Geometry: final body of the model. Coordinates: model frame, mm. Give positions to 0.01 mm unless a question says otherwise; leave off trailing zeros. Order: outer loops, then holes, each group sorted by start corner. A loop starts at its lowest first (then second) coordinate and runs counter-clockwise, first axis right, second up. Notation, with made-up numbers: (54, 9) -> (64, 9) arc R14 cw to (64, 24) -> close; hole circle Ø1 at (-5, 83.25). An arc over 180 degrees is marked (long way). Write item = value, one per line.
Autodesk Inventor part; units mm, degrees
ref_plane "Work Plane1" through (5, 2.5, 0) normal (0, 1, 0) x (-1, 0, 0)
ref_plane "YZ Plane" through (0, 0, 0) normal (1, 0, 0) x (0, 1, 0)
ref_plane "XY Plane" through (0, 0, 0) normal (0, 0, 1) x (1, 0, 0)
sketch "Sketch1" plane through (0, 0, 0) normal (0, 0, 1) x (1, 0, 0)
  line L0 (0, 0) -> (51.053, 0) construction
  line L1 (0, 0) -> (0, 2.5)
  line L2 (0, 2.5) -> (10, 2.5)
  line L3 (10, 2.5) -> (10, 4)
  line L4 (10, 4) -> (22, 4)
  line L5 (22, 4) -> (22, 0)
  line L6 (22, 0) -> (0, 0)
  dimension "d0" = 5
  dimension "d1" = 8
  dimension "d2" = 10
  dimension "d3" = 12
revolve "Revolution1" add sketch "Sketch1" angle 360 about axis through (0, 0, 0) along (1, 0, 0)
sketch "Sketch2" plane through (22, 0, 0) normal (1, 0, 0) x (0, 0, -1)
  circle A0 centre (0, 0) radius 4
  circle A1 centre (0, 0) radius 2.5 construction
  line L0 (-2.6458, 3) -> (2.6458, 3)
  arc A2 (2.6458, 3) -> (-2.6458, 3) centre (0, 0) ccw
  dimension "d5" = 3
extrude "Extrusion1" cut sketch "Sketch2" against normal through all contours L0 A0 picked at (-0.6179, 3.1815)
ref_plane "Work Plane1" through (5, 2.5, 0) normal (0, 1, 0) x (-1, 0, 0)
sketch "Sketch3" plane through (5, 2.5, 0) normal (0, 1, 0) x (-1, 0, 0)
  line L0 (-5, 2.5) -> (-5, -2.5) construction
  line L1 (5, 2.5) -> (5, -2.5) construction
  line L2 (-5, 2.6458) -> (-5, -2.6458) construction
  line L3 (-5, 0) -> (5, 0) construction
  point P0 (-1, 0)
  dimension "d8" = 4
hole "Hole1" at (6, 2.5, 0) direction (0, -1, 0) diameter 2 end through all
chamfer "Chamfer1" distance 1 angle 30 1 edges at (0, -2.5, 0) measured on face at (5.3098, -2.0345, -1.4529)
properties part number "P12" material "Aluminium"
1) Section query C-C (x = 4.75). Output: boundary loops of the cut face in (y, z).
Check sheet entries:
outline = circle Ø5 at (0, 0)
2) Section query D-D (y = -3.5). Output: boundary loops of the cut face in (x, z).
Check sheet entries:
outline = (10, -1.94) -> (22, -1.94) -> (22, 1.94) -> (10, 1.94) -> close
3) Mould query, pull axis Z, two halves, no side actions, for faces 1 (the face through (5, 0, 0)), 2 (the face through (10, -2, -2)), 3 (the face through (5.56, -0.54, -2.44)). Classes: +Z half, -Z half, draft (parallel to the pull), parting line (faces both ways), or undercut.
Check sheet entries:
face_1 = undercut
face_2 = draft
face_3 = parting line
4) Section query A-A (y = 0). Output: boundary loops of the cut face in (x, z), plus the area to 3 significant figures.
Check sheet entries:
outline = (0, -1.92) -> (1, -2.5) -> (10, -2.5) -> (10, -4) -> (22, -4) -> (22, 4) -> (10, 4) -> (10, 2.5) -> (1, 2.5) -> (0, 1.92) -> close; hole circle Ø2 at (6, 0)
area = 142 mm²
5) Section query B-B (z = 0). Output: boundary loops of the cut face in (x, y), plus the area to 3 significant figures.
Check sheet entries:
outline = (0, -1.92) -> (1, -2.5) -> (5, -2.5) -> (5, 2.5) -> (1, 2.5) -> (0, 1.92) -> close; (7, -2.5) -> (10, -2.5) -> (10, -4) -> (22, -4) -> (22, 3) -> (10, 3) -> (10, 2.5) -> (7, 2.5) -> close
area = 123 mm²
6) Line query: line 1 (X direction, y = 0.6, z = 0); line 2 (X direction, y = -1, z = -2.5); line 3 (Z direction, x = 6, y = -0.1). Output: solid intervals per line, ascending. Write a range as from..to.
Check sheet entries:
line_1 = 0..5, 7..22
line_2 = 10..22
line_3 = -2.5..-1, 1..2.5
7) First-contact query: P1, Ø1.5, axis at x = 8, z = -2.5, coming from the -Y side; P2, Ø1.6, axis at x = 6, z = 0, coming from the +Y side. Flat tips, straight axial feed; report the tip coordinate or a pass-through.
Check sheet entries:
P1 = -1.79
P2 = through
